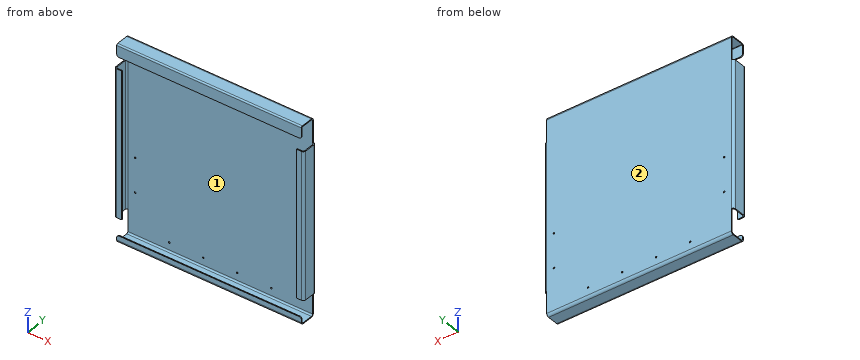
```python
from build123d import *

# Parameters (mm, degrees)
SKETCH1_W                     = 380
SKETCH1_H                     = 390
BASE_FLANGE1_DEPTH            = 2
EDGE_FLANGE3_DEPTH            = 380
EDGE_FLANGE11_DEPTH           = 380
EDGE_FLANGE12_STRIP_W         = 14
EDGE_FLANGE12_STRIP_H         = 2
EDGE_FLANGE12_STRIP_CUT_DEPTH = 380
EDGE_FLANGE12_DEPTH           = 380
EDGE_FLANGE13_STRIP_W         = 9.4732
EDGE_FLANGE13_STRIP_H         = 2
EDGE_FLANGE13_STRIP_CUT_DEPTH = 380
EDGE_FLANGE13_DEPTH           = 380
F_1_0MM_DOWEL_HOLE2_D         = 3.2
FILLET1_R                     = 5
EDGE_FLANGE14_DEPTH           = 300
EDGE_FLANGE15_DEPTH           = 300
EDGE_FLANGE16_STRIP_W         = 14
EDGE_FLANGE16_STRIP_H         = 2
EDGE_FLANGE16_STRIP_CUT_DEPTH = 300
EDGE_FLANGE16_DEPTH           = 300
EDGE_FLANGE17_STRIP_W         = 14
EDGE_FLANGE17_STRIP_H         = 2
EDGE_FLANGE17_STRIP_CUT_DEPTH = 300
EDGE_FLANGE17_DEPTH           = 300


# Sheet-metal steps are written as plain solids
with BuildPart() as part:
    # Sketch1 → Base-Flange1 (new body)
    with BuildSketch(Plane(origin=(0, 0, 0), x_dir=(1, 0, 0), z_dir=(0, 1, 0))):
        Rectangle(SKETCH1_W, SKETCH1_H)
    extrude(amount=-BASE_FLANGE1_DEPTH)

    # Edge-Flange3 section (across the edge) → Edge-Flange3 (add)
    with BuildSketch(Plane(origin=(-190, -2, -198), x_dir=(0, 0, 1), z_dir=(1, 0, 0))):
        with BuildLine():
            Line((-2, 3), (-2, 28))
            Line((-2, 28), (0, 28))
            Line((0, 28), (0, 3))
            ThreePointArc((0, 3), (0.878679656, 0.878679656), (3, 0))
            Line((3, 0), (3, -2))
            ThreePointArc((3, -2), (-0.535533906, -0.535533906), (-2, 3))
        make_face()
    extrude(amount=EDGE_FLANGE3_DEPTH)

    # Edge-Flange11 section (across the edge) → Edge-Flange11 (add)
    with BuildSketch(Plane(origin=(190, -2, 198), x_dir=(0, 0, -1), z_dir=(-1, 0, 0))):
        with BuildLine():
            Line((-2, 3), (-2, 28))
            Line((-2, 28), (0, 28))
            Line((0, 28), (0, 3))
            ThreePointArc((0, 3), (0.878679656, 0.878679656), (3, 0))
            Line((3, 0), (3, -2))
            ThreePointArc((3, -2), (-0.535533906, -0.535533906), (-2, 3))
        make_face()
    extrude(amount=EDGE_FLANGE11_DEPTH)

    # Edge-Flange12 strip (across the edge) → Edge-Flange12 strip cut (cut)
    with BuildSketch(Plane(origin=(-190, -30, -198), x_dir=(0, 1, 0), z_dir=(1, 0, 0))):
        with Locations((-4, -1)):
            Rectangle(EDGE_FLANGE12_STRIP_W, EDGE_FLANGE12_STRIP_H)
    extrude(amount=EDGE_FLANGE12_STRIP_CUT_DEPTH, mode=Mode.SUBTRACT)

    # Edge-Flange12 section (across the edge) → Edge-Flange12 (add)
    with BuildSketch(Plane(origin=(-190, -30, -198), x_dir=(0, 1, 0), z_dir=(1, 0, 0))):
        with BuildLine():
            Line((-2, 3), (-2, 13))
            Line((-2, 13), (0, 13))
            Line((0, 13), (0, 3))
            ThreePointArc((0, 3), (0.878679656, 0.878679656), (3, 0))
            Line((3, 0), (3, -2))
            ThreePointArc((3, -2), (-0.535533906, -0.535533906), (-2, 3))
        make_face()
    extrude(amount=EDGE_FLANGE12_DEPTH)

    # Edge-Flange13 strip (across the edge) → Edge-Flange13 strip cut (cut)
    with BuildSketch(Plane(origin=(190, -30, 198), x_dir=(0, 1, 0), z_dir=(-1, 0, 0))):
        with Locations((-4, -1)):
            Rectangle(EDGE_FLANGE13_STRIP_W, EDGE_FLANGE13_STRIP_H)
    extrude(amount=EDGE_FLANGE13_STRIP_CUT_DEPTH, mode=Mode.SUBTRACT)

    # Edge-Flange13 section (across the edge) → Edge-Flange13 (add)
    with BuildSketch(Plane(origin=(190, -30, 198), x_dir=(0, 1, 0), z_dir=(-1, 0, 0))):
        with BuildLine():
            Line((-2, 0.7366), (-2, 23))
            Line((-2, 23), (0, 23))
            Line((0, 23), (0, 0.7366))
            ThreePointArc((0, 0.7366), (0.215745145, 0.215745145), (0.7366, 0))
            Line((0.7366, 0), (0.7366, -2))
            ThreePointArc((0.7366, -2), (-1.198468417, -1.198468417), (-2, 0.7366))
        make_face()
    extrude(amount=EDGE_FLANGE13_DEPTH)

    # Ø1.0mm Dowel Hole2 (through all)
    with Locations(Plane(origin=(0, 0, 0), x_dir=(1, 0, 0), z_dir=(0, 1, 0))):
        with Locations((-175, 40), (-175, 110), (-105, 180), (-35, 180), (35, 180), (175, 110), (175, 40), (105, 180)):
            Hole(F_1_0MM_DOWEL_HOLE2_D / 2)

    # Fillet1
    fillet1_edges = [part.edges().sort_by_distance(p)[0] for p in [
        (190, -31, 175),
        (-190, -31, 175),
        (-190, -31, -185),
        (190, -31, -185),
    ]]
    fillet(fillet1_edges, radius=FILLET1_R)

    # Edge-Flange14 section (across the edge) → Edge-Flange14 (add)
    with BuildSketch(Plane(origin=(193, -2, -150), x_dir=(-1, 0, 0), z_dir=(0, 0, 1))):
        with BuildLine():
            Line((-2, 3), (-2, 30))
            Line((-2, 30), (0, 30))
            Line((0, 30), (0, 3))
            ThreePointArc((0, 3), (0.878679656, 0.878679656), (3, 0))
            Line((3, 0), (3, -2))
            ThreePointArc((3, -2), (-0.535533906, -0.535533906), (-2, 3))
        make_face()
    extrude(amount=EDGE_FLANGE14_DEPTH)

    # Edge-Flange15 section (across the edge) → Edge-Flange15 (add)
    with BuildSketch(Plane(origin=(-193, -2, 150), x_dir=(1, 0, 0), z_dir=(0, 0, -1))):
        with BuildLine():
            Line((-2, 3), (-2, 30))
            Line((-2, 30), (0, 30))
            Line((0, 30), (0, 3))
            ThreePointArc((0, 3), (0.878679656, 0.878679656), (3, 0))
            Line((3, 0), (3, -2))
            ThreePointArc((3, -2), (-0.535533906, -0.535533906), (-2, 3))
        make_face()
    extrude(amount=EDGE_FLANGE15_DEPTH)

    # Edge-Flange16 strip (across the edge) → Edge-Flange16 strip cut (cut)
    with BuildSketch(Plane(origin=(193, -32, -150), x_dir=(0, 1, 0), z_dir=(0, 0, 1))):
        with Locations((-2, -1)):
            Rectangle(EDGE_FLANGE16_STRIP_W, EDGE_FLANGE16_STRIP_H)
    extrude(amount=EDGE_FLANGE16_STRIP_CUT_DEPTH, mode=Mode.SUBTRACT)

    # Edge-Flange16 section (across the edge) → Edge-Flange16 (add)
    with BuildSketch(Plane(origin=(193, -32, -150), x_dir=(0, 1, 0), z_dir=(0, 0, 1))):
        with BuildLine():
            Line((0, 3), (0, 13))
            Line((0, 13), (2, 13))
            Line((2, 13), (2, 3))
            ThreePointArc((2, 3), (2.878679656, 0.878679656), (5, 0))
            Line((5, 0), (5, -2))
            ThreePointArc((5, -2), (1.464466094, -0.535533906), (0, 3))
        make_face()
    extrude(amount=EDGE_FLANGE16_DEPTH)

    # Edge-Flange17 strip (across the edge) → Edge-Flange17 strip cut (cut)
    with BuildSketch(Plane(origin=(-193, -32, 150), x_dir=(0, 1, 0), z_dir=(0, 0, -1))):
        with Locations((-2, -1)):
            Rectangle(EDGE_FLANGE17_STRIP_W, EDGE_FLANGE17_STRIP_H)
    extrude(amount=EDGE_FLANGE17_STRIP_CUT_DEPTH, mode=Mode.SUBTRACT)

    # Edge-Flange17 section (across the edge) → Edge-Flange17 (add)
    with BuildSketch(Plane(origin=(-193, -32, 150), x_dir=(0, 1, 0), z_dir=(0, 0, -1))):
        with BuildLine():
            Line((0, 3), (0, 13))
            Line((0, 13), (2, 13))
            Line((2, 13), (2, 3))
            ThreePointArc((2, 3), (2.878679656, 0.878679656), (5, 0))
            Line((5, 0), (5, -2))
            ThreePointArc((5, -2), (1.464466094, -0.535533906), (0, 3))
        make_face()
    extrude(amount=EDGE_FLANGE17_DEPTH)


solid = part.part
```
Work out the finished part from the listing and answer in its coordinate system (mm). Face numbers are marked on the shaded views. Round coordinates to 2 decimals unless told otherwise and drop trailing zeros. Write each loop counter-clockwise with the first axis right and the second up, starting at its lowest first coordinate (ties: lowest second). Pieces come first, ordered by that corner, then holes.
1) A cutting plane is placed at A-A on y = -18. Determine the outline of the cut face in (x, z).
2) A cutting plane is placed at B-B on x = -128. Determine the outline of the cut face in (y, z), and give its area (3 significant figures).
3) A cutting plane is placed at C-C on z = 88. Determine the outline of the cut face in (x, y), and give its area (3 significant figures).
4) A cutting plane is placed at D-D on z = -165. Determine the outline of the cut face in (x, y), and give its area (3 significant figures).
5) Flat-ended cylindrical pins translate along their axes: P1, Ø1.6, axis at x = 71, y = -30.5, coming from the +Z side; P2, Ø4, axis at x = -175, z = -40, coming from the -Y side; P3, Ø2, axis at y = -30.5, z = 70.5, coming from the -X side; P4, Ø11, axis at x = 14, z = 189, coming from the +Y side. Find the tip coordinate at first contact, or state that the pin passes through.
6) Determine the mould class of the marked faces 1 and 2 for opening direction Z: pulls with the +Z half, pulls with the -Z half, needs draft (parallel to the pull), parting line crosses it, or undercut.
7) Consider probe 1 along X at (y, z) = (-1, -180); probe 2 along Z at (x, y) = (175, -1); probe 3 along X at (y, z) = (-1, -110). Determine where each line is inside the solid, lowest interval first.
Entries:
1. outline: (-195, -150) - (-193, -150) - (-193, 150) - (-195, 150) - close; (-190, -200) - (190, -200) - (190, -198) - (-190, -198) - close; (-190, 198) - (190, 198) - (190, 200) - (-190, 200) - close; (193, -150) - (195, -150) - (195, 150) - (193, 150) - close
2. outline: (-32, -195) arc R5 ccw to (-27, -200) - (-5, -200) arc R5 ccw to (0, -195) - (0, 195) arc R5 ccw to (-5, 200) - (-29.26, 200) arc R2.74 ccw to (-32, 197.26) - (-32, 175) - (-30, 175) - (-30, 197.26) arc R0.74 cw to (-29.26, 198) - (-5, 198) arc R3 cw to (-2, 195) - (-2, -195) arc R3 cw to (-5, -198) - (-27, -198) arc R3 cw to (-30, -195) - (-30, -185) - (-32, -185) - close
2. area: 980 mm2
3. outline: (-195, -27) arc R5 ccw to (-190, -32) - (-180, -32) - (-180, -30) - (-190, -30) arc R3 cw to (-193, -27) - (-193, -5) arc R3 cw to (-190, -2) - (190, -2) arc R3 cw to (193, -5) - (193, -27) arc R3 cw to (190, -30) - (180, -30) - (180, -32) - (190, -32) arc R5 ccw to (195, -27) - (195, -5) arc R5 ccw to (190, 0) - (-190, 0) arc R5 ccw to (-195, -5) - close
3. area: 938 mm2
4. outline: (-190, -2) - (190, -2) - (190, 0) - (-190, 0) - close
4. area: 760 mm2
5. P1: stops at z = 199.96
5. P2: stops at y = -2
5. P3: stops at x = -194.33
5. P4: stops at y = 0
6. face 1: undercut
6. face 2: needs draft
7. probe 1: x = -190 to -106.6, -103.4 to -36.6, -33.4 to 33.4, 36.6 to 103.4, 106.6 to 190
7. probe 2: z = -198 to -111.6, -108.4 to -41.6, -38.4 to 198
7. probe 3: x = -193 to -176.6, -173.4 to 173.4, 176.6 to 193
